```python
from build123d import *
from OCP.BRepFilletAPI import BRepFilletAPI_MakeChamfer

# Parameters (mm, degrees)
BOSS_EXTRUDE1_DEPTH = 15
SKETCH4_W           = 106
SKETCH4_H           = 57
BOSS_EXTRUDE3_DEPTH = 40
SKETCH5_W           = 25.4
SKETCH5_H           = 12.7
CUT_EXTRUDE3_DEPTH  = 12
SKETCH5_3_W         = 25.4
SKETCH5_3_H         = 27.3
CUT_EXTRUDE4_DEPTH  = 88.509999429
CHAMFER3_SIZE       = 45
CHAMFER3_SIZE2      = 30
FILLET2_R           = 3


with BuildPart() as part:
    # Sketch1 → Boss-Extrude1 (new body)
    with BuildSketch(Plane.XY):
        Polygon((23, -13.5), (53, -13.5), (53, 43.5), (-53, 43.5), (-53, -13.5), (-23, -13.5), (-23, 13.5), (23, 13.5), align=None)
    extrude(amount=BOSS_EXTRUDE1_DEPTH)

    # Chamfer1
    # the kernel refuses this chamfer: 30, 15 mm, written as the material it takes off along each edge
    with BuildSketch(Plane(origin=(23, 13.5, 15), x_dir=(-0.06891834360170887, 0, -0.9976223042390325), z_dir=(0, -1, 0)), Plane(origin=(-23, -13.5, 15), x_dir=(0.06891834360170887, 0, -0.9976223042390325), z_dir=(0, 1, 0))) as chamfer1_piece_1:
        with BuildLine():
            Line((15.573685801, 0), (-2.676901546, 30.962444281))
            Line((-2.676901546, 30.962444281), (-3.275474928, 30.921093275))
            ThreePointArc((-3.275474928, 30.921093275), (-1.669334001, 15.458363867), (-0.598573383, -0.041351006))
            Line((-0.598573383, -0.041351006), (0.041351006, -0.598573383))
            ThreePointArc((0.041351006, -0.598573383), (7.791208443, -0.063193073), (15.615036807, -0.598573383))
            Line((15.615036807, -0.598573383), (15.573685801, 0))
        make_face()
    extrude(amount=27, mode=Mode.SUBTRACT)
    with BuildSketch(Plane(origin=(-23, 13.5, 15), x_dir=(0, -0.06891834360170876, -0.9976223042390325), z_dir=(1, 0, 0))) as chamfer1_piece_2:
        with BuildLine():
            Line((15.573685801, 0), (-2.676901546, 30.962444281))
            Line((-2.676901546, 30.962444281), (-3.275474928, 30.921093275))
            ThreePointArc((-3.275474928, 30.921093275), (-1.669334001, 15.458363867), (-0.598573383, -0.041351006))
            Line((-0.598573383, -0.041351006), (0.041351006, -0.598573383))
            ThreePointArc((0.041351006, -0.598573383), (7.791208443, -0.063193073), (15.615036807, -0.598573383))
            Line((15.615036807, -0.598573383), (15.573685801, 0))
        make_face()
    extrude(amount=46, mode=Mode.SUBTRACT)
    with BuildSketch(Plane(origin=(-23, 13.5, 15), x_dir=(0, -0.06891834360170876, -0.9976223042390325), z_dir=(1, 0, 0))) as chamfer1_piece_3a_section:
        with BuildLine():
            Line((15.573685801, 0), (-2.676901546, 30.962444281))
            Line((-2.676901546, 30.962444281), (-3.275474928, 30.921093275))
            ThreePointArc((-3.275474928, 30.921093275), (-1.669334001, 15.458363867), (-0.598573383, -0.041351006))
            Line((-0.598573383, -0.041351006), (0.041351006, -0.598573383))
            ThreePointArc((0.041351006, -0.598573383), (7.791208443, -0.063193073), (15.615036807, -0.598573383))
            Line((15.615036807, -0.598573383), (15.573685801, 0))
        make_face()
    chamfer1_piece_3a = extrude(amount=123.694866214, mode=Mode.PRIVATE)
    chamfer1_piece_3a = split(chamfer1_piece_3a, bisect_by=Plane(origin=(23, 23.617605247, 10.241766787), z_dir=(1, 0, 0)), keep=Keep.TOP, mode=Mode.PRIVATE)
    with BuildSketch(Plane(origin=(23, 91.194866214, 15), x_dir=(-0.06891834360170887, 0, -0.9976223042390325), z_dir=(0, -1, 0))) as chamfer1_piece_3b_section:
        with BuildLine():
            Line((15.573685801, 0), (-2.676901546, 30.962444281))
            Line((-2.676901546, 30.962444281), (-3.275474928, 30.921093275))
            ThreePointArc((-3.275474928, 30.921093275), (-1.669334001, 15.458363867), (-0.598573383, -0.041351006))
            Line((-0.598573383, -0.041351006), (0.041351006, -0.598573383))
            ThreePointArc((0.041351006, -0.598573383), (7.791208443, -0.063193073), (15.615036807, -0.598573383))
            Line((15.615036807, -0.598573383), (15.573685801, 0))
        make_face()
    chamfer1_piece_3b = extrude(amount=104.694866214, mode=Mode.PRIVATE)
    chamfer1_piece_3b = split(chamfer1_piece_3b, bisect_by=Plane(origin=(33.117605247, 13.5, 10.241766787), z_dir=(0, 1, 0)), keep=Keep.TOP, mode=Mode.PRIVATE)
    chamfer1_piece_3 = chamfer1_piece_3a & chamfer1_piece_3b
    add(chamfer1_piece_3, mode=Mode.SUBTRACT)
    with BuildSketch(Plane(origin=(-23, -13.5, 15), x_dir=(0.06891834360170887, 0, -0.9976223042390325), z_dir=(0, 1, 0))) as chamfer1_piece_4a_section:
        with BuildLine():
            Line((15.573685801, 0), (-2.676901546, 30.962444281))
            Line((-2.676901546, 30.962444281), (-3.275474928, 30.921093275))
            ThreePointArc((-3.275474928, 30.921093275), (-1.669334001, 15.458363867), (-0.598573383, -0.041351006))
            Line((-0.598573383, -0.041351006), (0.041351006, -0.598573383))
            ThreePointArc((0.041351006, -0.598573383), (7.791208443, -0.063193073), (15.615036807, -0.598573383))
            Line((15.615036807, -0.598573383), (15.573685801, 0))
        make_face()
    chamfer1_piece_4a = extrude(amount=104.694866214, mode=Mode.PRIVATE)
    chamfer1_piece_4a = split(chamfer1_piece_4a, bisect_by=Plane(origin=(-33.117605247, 13.5, 10.241766787), z_dir=(0, 1, 0)), keep=Keep.TOP, mode=Mode.PRIVATE)
    with BuildSketch(Plane(origin=(-100.694866214, 13.5, 15), x_dir=(0, -0.06891834360170876, -0.9976223042390325), z_dir=(1, 0, 0))) as chamfer1_piece_4b_section:
        with BuildLine():
            Line((15.573685801, 0), (-2.676901546, 30.962444281))
            Line((-2.676901546, 30.962444281), (-3.275474928, 30.921093275))
            ThreePointArc((-3.275474928, 30.921093275), (-1.669334001, 15.458363867), (-0.598573383, -0.041351006))
            Line((-0.598573383, -0.041351006), (0.041351006, -0.598573383))
            ThreePointArc((0.041351006, -0.598573383), (7.791208443, -0.063193073), (15.615036807, -0.598573383))
            Line((15.615036807, -0.598573383), (15.573685801, 0))
        make_face()
    chamfer1_piece_4b = extrude(amount=123.694866214, mode=Mode.PRIVATE)
    chamfer1_piece_4b = split(chamfer1_piece_4b, bisect_by=Plane(origin=(-23, 23.617605247, 10.241766787), z_dir=(-1, 0, 0)), keep=Keep.TOP, mode=Mode.PRIVATE)
    chamfer1_piece_4 = chamfer1_piece_4a & chamfer1_piece_4b
    add(chamfer1_piece_4, mode=Mode.SUBTRACT)

    # Sketch4 → Boss-Extrude3 (add)
    with BuildSketch(Plane(origin=(0, 0, 0), x_dir=(-1, 0, 0), z_dir=(0, 0, -1))):
        with Locations((0, 15)):
            Rectangle(SKETCH4_W, SKETCH4_H)
    extrude(amount=BOSS_EXTRUDE3_DEPTH)

    # Sketch5 → Cut-Extrude3 (cut)
    with BuildSketch(Plane.XZ.offset(13.5)):
        with Locations((0, -6.35)):
            Rectangle(SKETCH5_W, SKETCH5_H)
    extrude(amount=-CUT_EXTRUDE3_DEPTH, mode=Mode.SUBTRACT)

    # Sketch5<3> → Cut-Extrude4 (cut, through all)
    with BuildSketch(Plane.XZ.offset(13.5)):
        with Locations((0, -26.35)):
            Rectangle(SKETCH5_3_W, SKETCH5_3_H)
    extrude(amount=-CUT_EXTRUDE4_DEPTH, mode=Mode.SUBTRACT)

    # Chamfer3: one chamfer whose edges measure the first distance from different faces: ONE call of the kernel's chamfer builder (chamfer() names one face for all edges)
    chamfer3_edges_1 = [part.edges().sort_by_distance(p)[0] for p in [
        (53, 15, -40),
    ]]
    chamfer3_side_1 = [part.faces().sort_by_distance(p)[0] for p in [
        (53, 15, -12.5),
    ]]
    chamfer3_edges_2 = [part.edges().sort_by_distance(p)[0] for p in [
        (-53, 15, -40),
    ]]
    chamfer3_side_2 = [part.faces().sort_by_distance(p)[0] for p in [
        (-53, 15, -12.5),
    ]]
    chamfer3 = BRepFilletAPI_MakeChamfer(part.part.solid().wrapped)
    for e in chamfer3_edges_1:
        chamfer3.Add(CHAMFER3_SIZE, CHAMFER3_SIZE2, e.wrapped, chamfer3_side_1[0].wrapped)  # the first distance lies on this face
    for e in chamfer3_edges_2:
        chamfer3.Add(CHAMFER3_SIZE, CHAMFER3_SIZE2, e.wrapped, chamfer3_side_2[0].wrapped)  # the first distance lies on this face
    add(Compound.cast(chamfer3.Shape()), mode=Mode.REPLACE)

    # Fillet2
    fillet2_edges = [part.edges().sort_by_distance(p)[0] for p in [
        (23, 0, 0),
        (0, 13.5, 0),
        (-23, 0, 0),
    ]]
    fillet(fillet2_edges, radius=FILLET2_R)
    fillet2_2_edges = [part.edges().sort_by_distance(p)[0] for p in [
        (53, 15, 15),
        (0, 43.5, 15),
        (-53, 15, 15),
        (38.316718427, -13.5, 7.658359213),
        (-38.316718427, -13.5, 7.658359213),
        (17.495898034, -13.5, 0),
        (-17.495898034, -13.5, 0),
        (-22.981054829, -13.5, 0.080253032),
        (22.981054829, -13.5, 0.080253032),
    ]]
    fillet(fillet2_2_edges, radius=FILLET2_R)


solid = part.part
```
Work out the finished part from the listing and answer in its coordinate system (mm). A direction names the side the tool comes from. Round coordinates to 2 decimals unless told otherwise and drop trailing zeros. Write each loop counter-clockwise with the first axis right and the second up, starting at its lowest first coordinate (ties: lowest second). Pieces come first, ordered by that corner, then holes.
1) A cutting plane is placed at A-A on z = -23.5. Determine the outline of the cut face in (x, y), and give its area (3 significant figures).
2) A cutting plane is placed at D-D on z = -8.5. Determine the outline of the cut face in (x, y).
3) Which of the six approach directions +Z, -Z, +X, -X, +Y, -Y give full straight-line access (tool end or side, diameter ignored) to faces 5 (the face through (0, 21, -12.7)), 6 (the face through (-53, 15, 8)), 7 (the face through (0, 4, 0))?
4) Consider probe 1 along X at (y, z) = (3, -37); probe 2 along Z at (x, y) = (13.5, -9); probe 3 along X at (y, z) = (38.5, -24). Determine where each line is inside the solid, lowest interval first.
5) Determine the mould class of faces 1 (the face through (53, 15, 8)), 2 (the face through (17.56, -12.6, -0.86)), 3 (the face through (-28, -13.5, -14)), 4 (the face through (-0.7, 29.3, 7.9)) for opening direction X: pulls with the +X half, pulls with the -X half, needs draft (parallel to the pull), parting line crosses it, or undercut.
6) A cutting plane is placed at C-C on x = -7.5. Determine the outline of the cut face in (y, z), and give its area (3 significant figures).
7) Flat-ended cylindrical pins translate along their axes: P1, Ø14, axis at x = -2, z = -8.5, coming from the -Y side; P2, Ø12, axis at y = 17, z = -6, coming from the -X side; P3, Ø11.5, axis at x = 1, y = 4, coming from the +Z side. Find the tip coordinate at first contact, or state that the pin passes through.
8) A cutting plane is placed at B-B on y = 19. Determine the outline of the cut face in (x, z), and give its area (3 significant figures).
Entries:
1. outline: (-34, -13.5) - (-12.7, -13.5) - (-12.7, 43.5) - (-34, 43.5) - close; (12.7, -13.5) - (34, -13.5) - (34, 43.5) - (12.7, 43.5) - close
1. area: 2,430 mm2
2. outline: (-44, -13.5) - (-12.7, -13.5) - (-12.7, -1.5) - (12.7, -1.5) - (12.7, -13.5) - (44, -13.5) - (44, 43.5) - (-44, 43.5) - close
3. face 5: -Z, +Y, -Y
3. face 6: +Z, -Z, -X, +Y, -Y
3. face 7: +Z, -Y
4. probe 1: x = -25 to -12.7, 12.7 to 25
4. probe 2: z = -40 to 0
4. probe 3: x = -33.67 to -12.7, 12.7 to 33.67
5. face 1: pulls with the +X half
5. face 2: undercut
5. face 3: needs draft
5. face 4: undercut
6. outline: (-1.5, -12.7) - (43.5, -12.7) - (43.5, 10.15) arc R3 ccw to (39.16, 12.83) - (14.13, 0.32) arc R3 cw to (12.79, 0) - (-1.5, 0) - close
6. area: 791 mm2
7. P1: stops at y = -1.5
7. P2: stops at x = -49.67
7. P3: stops at z = 0
8. outline: (-53, 5) - (-23, -40) - (-12.7, -40) - (-12.7, -12.7) - (12.7, -12.7) - (12.7, -40) - (23, -40) - (53, 5) - (53, 10.15) arc R3 ccw to (48.66, 12.83) - (28.5, 2.75) - (-28.5, 2.75) - (-48.66, 12.83) arc R3 ccw to (-53, 10.15) - close
8. area: 2,780 mm2
